from build123d import *

# Parameters (mm, degrees)
F1_DEPTH = 12.7
F2_R     = 18.3515
F3_DEPTH = 27.9908
F4_R     = 12.0015
F5_DEPTH = 40.6918
F6_D     = 8.3312
F7_R     = 2.3622
F8_DEPTH = 25.4


with BuildPart() as f1:
    # F0 (on Right) → F1 (new body)
    with BuildSketch(Plane.YZ):
        with BuildLine():
            Line((21.060567, 31.75), (-21.060567, 31.75))
            ThreePointArc((-21.060567, 31.75), (-38.1, 0), (-21.060567, -31.75))
            Line((-21.060567, -31.75), (21.060567, -31.75))
            ThreePointArc((21.060567, -31.75), (38.1, 0), (21.060567, 31.75))
        make_face()
    extrude(amount=-F1_DEPTH)

    # F2 (on face) → F3 (join)
    with BuildSketch(Plane(origin=(-12.7, 0, 0), x_dir=(0, -1, 0), z_dir=(-1, 0, 0))):
        Circle(F2_R)
    extrude(amount=F3_DEPTH)

    # F4 (on face) → F5 (cut, through all)
    with BuildSketch(Plane.YZ):
        Circle(F4_R)
    extrude(amount=-F5_DEPTH, mode=Mode.SUBTRACT)

    # F6 (through all)
    with Locations(Plane.YZ):
        with Locations((26.1874, 0), (-26.1874, 0)):
            Hole(F6_D / 2)

    # F7 (on Front) → F8 (cut)
    with BuildSketch(Plane.XZ):
        with Locations((-34.3408, 0)):
            Circle(F7_R)
    extrude(amount=-F8_DEPTH, mode=Mode.SUBTRACT)


solid = f1.part
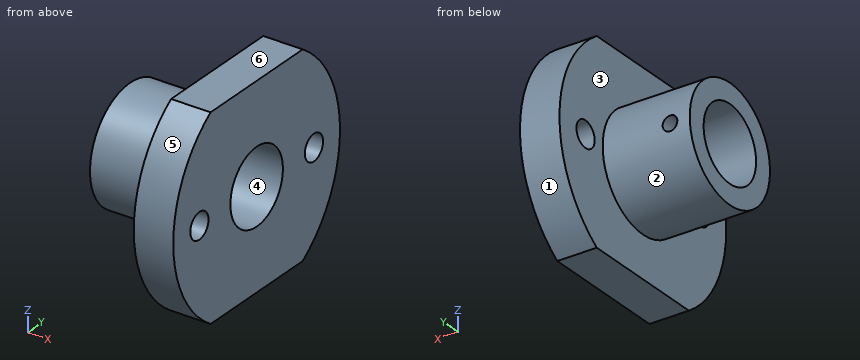
Geometry check sheet. Reference: the model listing, model coordinates, mm. Face numbers are marked on the shaded views. A direction names the side the tool comes from. Give positions to 0.01 mm unless a question says otherwise; leave off trailing zeros. Order: outer loops, then holes, each group sorted by start corner. A loop starts at its lowest first (then second) coordinate and runs counter-clockwise, first axis right, second up. Notation, with made-up numbers: (-11.5, -36.75) - (29.5, -36.75) arc R29 ccw to (29.5, -4.75) - close; hole circle Ø5 at (58, 74). An arc over 180 degrees is marked (long way). Use one line per item in the form item = value.
1) Material ranges on probe 1 along X at (y, z) = (15.5, 0); probe 2 along Z at (x, y) = (-12, 0); probe 3 along X at (y, z) = (-21.5, -26), recorded low to high. Write a range as from..to.
Working result:
probe_1 = -40.69..-36.7, -31.98..0
probe_2 = -31.75..-12, 12..31.75
probe_3 = -12.7..0
2) Sectioned sample at A-A (y = 0). Record the boundary of the cut face in (x, z).
Working result:
outline = (-40.69, -18.35) - (-12.7, -18.35) - (-12.7, -31.75) - (0, -31.75) - (0, -12) - (-40.69, -12) - close; (-40.69, 12) - (0, 12) - (0, 31.75) - (-12.7, 31.75) - (-12.7, 18.35) - (-40.69, 18.35) - close
3) Draft check along Z on the marked faces 3, 4, 5 and 6. Enter one of: released by +Z, released by -Z, zero draft, split by the parting line, or undercut.
Working result:
face_3 = zero draft
face_4 = undercut
face_5 = split by the parting line
face_6 = released by +Z
4) Sectioned sample at D-D (y = 17). Record the boundary of the cut face in (x, z).
Working result:
outline = (-40.69, -6.91) - (-12.7, -6.91) - (-12.7, -31.75) - (0, -31.75) - (0, 31.75) - (-12.7, 31.75) - (-12.7, 6.91) - (-40.69, 6.91) - close; hole circle Ø4.72 at (-34.34, 0)
5) Sectioned sample at B-B (z = 0). Record the boundary of the cut face in (x, y).
Working result:
outline = (-40.69, -18.35) - (-12.7, -18.35) - (-12.7, -22.02) - (0, -22.02) - (0, -12) - (-40.69, -12) - close; (-40.69, 12) - (-36.7, 12) - (-36.7, 18.35) - (-40.69, 18.35) - close; (-31.98, 12) - (0, 12) - (0, 22.02) - (-12.7, 22.02) - (-12.7, 18.35) - (-31.98, 18.35) - close; (-12.7, -38.1) - (0, -38.1) - (0, -30.35) - (-12.7, -30.35) - close; (-12.7, 30.35) - (0, 30.35) - (0, 38.1) - (-12.7, 38.1) - close
6) Sectioned sample at C-C (x = -1.5). Record the boundary of the cut face in (y, z), and give its area (3 significant figures).
Working result:
outline = (-21.06, -31.75) - (21.06, -31.75) arc R38.1 ccw to (21.06, 31.75) - (-21.06, 31.75) arc R38.1 ccw to start; hole circle Ø8.33 at (-26.19, 0); hole circle Ø24 at (0, 0); hole circle Ø8.33 at (26.19, 0)
area = 3,640 mm^2
7) Access from +Z, -Z, +X, -X, +Y, -Y to the whole of each face (thin tool, end or side, straight path). Record for the marked faces 1 and 2.
Working result:
face_1 = +X, -X, +Y
face_2 = -X
8) Depth check by flat-ended pin: pin 1 Ø12 at (x, z) = (-22, 9.5) entering from +Y; pin 2 Ø10 at (x, z) = (-22.5, -5.5) entering from +Y; pin 3 Ø10 at (x, z) = (-11, -20.5) entering from +Y; pin 4 Ø12 at (x, y) = (-8, 27) entering from -Z. Enter the tip coordinate at first touch or a pass-through.
Working result:
pin_1 = 18.01
pin_2 = 18.34
pin_3 = 34.8
pin_4 = -31.75
